CAD build for the part. Positions are in the model's coordinates, mm. A direction names the side the tool comes from. Give positions to 0.01 mm unless a question says otherwise; leave off trailing zeros. Write each loop counter-clockwise with the first axis right and the second up, starting at its lowest first coordinate (ties: lowest second). Pieces come first, ordered by that corner, then holes. Notation, with made-up numbers: (-35, -28.75) - (22, -28.75) arc R21 cw to (22, 0.25) - close; hole circle Ø3 at (-21.5, 32.5). An arc over 180 degrees is marked (long way). Answer as a JSON object with one key per item and string values.
from build123d import *

# Parameters (mm, degrees)
RESSALTO_EXTRUS_O1_DEPTH   = 50
ESBO_O3_W                  = 6
ESBO_O3_H                  = 17.5
CORTE_EXTRUS_O2_DEPTH      = 80
ESBO_O4_W                  = 20
ESBO_O4_H                  = 11.5
CORTE_EXTRUS_O3_DEPTH      = 18
ESBO_O5_R                  = 1.75
ESBO_O5_W                  = 3
ESBO_O5_H                  = 22.5
CORTE_EXTRUS_O4_DEPTH      = 90.5
CORTE_EXTRUS_O4_DEPTH_BACK = 4.5


with BuildPart() as part:
    # Esboço1 → Ressalto-extrusão1 (new body)
    with BuildSketch(Plane.XY):
        Polygon((21, 0), (0, 0), (0, 4), (-2, 1), (-3, 1), (-3, 4), (0, 8.5), (0, 93), (3, 93), (3, 13), (10.5, 5.5), (18, 13), (18, 15), (21, 15), align=None)
    extrude(amount=RESSALTO_EXTRUS_O1_DEPTH)

    # Esboço3 → Corte-extrusão2 (cut)
    with BuildSketch(Plane(origin=(0, 93, 0), x_dir=(1, 0, 0), z_dir=(0, 1, 0))):
        with Locations((0, -8.75)):
            Rectangle(ESBO_O3_W, ESBO_O3_H)
        with Locations((0, -41.25)):
            Rectangle(ESBO_O3_W, ESBO_O3_H)
    extrude(amount=-CORTE_EXTRUS_O2_DEPTH, mode=Mode.SUBTRACT)

    # Esboço4 → Corte-extrusão3 (cut)
    with BuildSketch(Plane(origin=(21, 0, 0), x_dir=(0, 0, -1), z_dir=(1, 0, 0))):
        with Locations((-25, 9.25)):
            Rectangle(ESBO_O4_W, ESBO_O4_H)
    extrude(amount=-CORTE_EXTRUS_O3_DEPTH, mode=Mode.SUBTRACT)

    # Esboço5 → Corte-extrusão4 (cut, two sides)
    with BuildSketch(Plane(origin=(0, 3.5, 0), x_dir=(1, 0, 0), z_dir=(0, 1, 0))) as corte_extrus_o4_sk:
        with Locations((10.5, -20)):
            Circle(ESBO_O5_R)
        with Locations((10.5, -30)):
            Circle(ESBO_O5_R)
        with Locations((-1.5, -11.25)):
            Rectangle(ESBO_O5_W, ESBO_O5_H)
        with Locations((-1.5, -38.75)):
            Rectangle(ESBO_O5_W, ESBO_O5_H)
    extrude(amount=CORTE_EXTRUS_O4_DEPTH, mode=Mode.SUBTRACT)
    extrude(corte_extrus_o4_sk.sketch, amount=-CORTE_EXTRUS_O4_DEPTH_BACK, mode=Mode.SUBTRACT)


solid = part.part
Item 1: Cut at C-C (y = 45.5). Give the cut face in (x, z), and give its area (3 significant figures).
Entries:
{"outline": "(0, 17.5) - (3, 17.5) - (3, 32.5) - (0, 32.5) - close", "area": "45.0 mm2"}
Item 2: Which spindle directions (+Z, -Z, +X, -X, +Y, -Y) get a long thin tool onto all of the face, cutting with end or side? Do faces 1 (the flat face through (18, 14, 7)), 2 (the flat face through (-2, 4, 22.5)), 3 (the flat face through (7, 9, 7)), 4 (the flat face through (1, 13, 9)). Say none if no direction does.
Entries:
{"face 1": "+Z, -Z, -X, +Y", "face 2": "-Z, -X, +Y, -Y", "face 3": "+Z, -Z, +Y", "face 4": "-Z, -X, +Y"}
Item 3: Cut at B-B (x = 15.5). Give the cut face in (y, z), and give its area (3 significant figures).
Entries:
{"outline": "(0, 0) - (10.5, 0) - (10.5, 15) - (3.5, 15) - (3.5, 35) - (10.5, 35) - (10.5, 50) - (0, 50) - close", "area": "385 mm2"}
Item 4: Flat gauge pins, fed straight in: P1, Ø0.9, axis at x = 1, z = 45, coming from the +Y side; P2, Ø1.6, axis at y = 13.5, z = 8, coming from the -X side; P3, Ø1.5, axis at x = -2, y = 3, coming from the +Z side. Where does each tip first touch, or does it go through?
Entries:
{"P1": "y = 13", "P2": "x = 0", "P3": "z = 27.5"}
Item 5: Cut at D-D (z = 4.5). Give the cut face in (x, y), and give its area (3 significant figures).
Entries:
{"outline": "(0, 0) - (21, 0) - (21, 15) - (18, 15) - (18, 13) - (10.5, 5.5) - (3, 13) - (0, 13) - close", "area": "223 mm2"}
Item 6: Mould opens along X. For faces 5 (the flat face through (1, 54, 32.5)), 6 (the cylindrical face through (10.272, 1.774, 18.265)), 7 (the flat face through (-1.52, 6.22, 24.96)) say: +X half, -X half, draft (parallel to the pull), parting line (faces both ways), or undercut.
Entries:
{"face 5": "draft", "face 6": "undercut", "face 7": "-X half"}
Item 7: Probe line 1 (Z direction, x = 10.5, y = 1.25); line 2 (X direction, y = 2, z = 20); line 3 (Y direction, x = 15.25, z = 18). List the from-to ranges inside material, lowest first. Write a range as from..to.
Entries:
{"line 1": "0..18.25, 21.75..28.25, 31.75..50", "line 2": "0..8.75, 12.25..21", "line 3": "0..3.5"}
Item 8: Cut at A-A (z = 20). Give the cut face in (x, y), and give its area (3 significant figures).
Entries:
{"outline": "(0, 0) - (8.75, 0) - (8.75, 3.5) - (3, 3.5) - (3, 93) - (0, 93) - close; (12.25, 0) - (21, 0) - (21, 3.5) - (12.25, 3.5) - close", "area": "330 mm2"}
